Can you work these out from the model? Positions are in its coordinate system, mm. A direction names the side the tool comes from. Round coordinates to 2 decimals unless told otherwise and drop trailing zeros. Loops run counter-clockwise (first coordinate to the right, second up) from the corner with the lowest first, then second, coordinate; pieces in that order, holes last. Notation, with made-up numbers: M -25,80.25 L -17,80.25 A14 cw -17,89.25 Z; hole C 74,-2.5 d2. An arc over 180 degrees is marked long. Return JSON: item names as keys, results as strings.
```python
from build123d import *

# Parameters (mm, degrees)
SKETCH_1_R          = 1.55
EXTRUDE_1_DEPTH     = 3
CUT_EXTRUDE_1_DEPTH = 1
CHAMFER_1_SIZE      = 0.3


with BuildPart() as part:
    # 草图1 → 凸台-拉伸1 (new body)
    with BuildSketch(Plane(origin=(0, 0, 0), x_dir=(-1, 0, 0), z_dir=(0, 0, -1))):
        with BuildLine():
            Line((-47.519320255, 26.959319012), (-50.6992, 14.4996))
            Line((-50.6992, 14.4996), (-50.6992, 10.0003))
            Line((-50.6992, 10.0003), (-53.6992, 10.0003))
            Line((-53.6992, 10.0003), (-53.6992, 0))
            Line((-53.6992, 0), (-50.6992, 0))
            Line((-50.6992, 0), (-50.6992, -1.5007))
            Line((-50.6992, -1.5007), (-49.2382, -1.5007))
            Line((-49.2382, -1.5007), (-49.2382, -4.5007))
            Line((-49.2382, -4.5007), (-40.2392, -4.5007))
            Line((-40.2392, -4.5007), (-40.2392, -1.4993))
            Line((-40.2392, -1.4993), (-34.2002, -1.4993))
            Line((-34.2002, -1.4993), (-34.2002, 1.0005))
            Line((-34.2002, 1.0005), (-19.2003, 1.0005))
            Line((-19.2003, 1.0005), (-19.2003, -1.4993))
            Line((-19.2003, -1.4993), (-11.7217, -1.4993))
            Line((-11.7217, -1.4993), (-11.7217, -4.5007))
            Line((-11.7217, -4.5007), (-4.3215, -4.5007))
            Line((-4.3215, -4.5007), (-4.3215, -1.5007))
            Line((-4.3215, -1.5007), (-3, -1.5007))
            Line((-3, -1.5007), (-3, 0))
            Line((-3, 0), (0, 0))
            Line((0, 0), (0, 10.0003))
            Line((0, 10.0003), (-3, 10.0003))
            Line((-3, 10.0003), (-3, 14.4996))
            Line((-3, 14.4996), (-26.543543046, 20.807804388))
            ThreePointArc((-26.543543046, 20.807804388), (-32.65852857, 22.990550509), (-36.548909006, 28.188854909))
            ThreePointArc((-36.548909006, 28.188854909), (-38.379715818, 30.572322748), (-41.246222879, 31.4756))
            Line((-41.246222879, 31.4756), (-41.70566582, 31.4756))
            ThreePointArc((-41.70566582, 31.4756), (-45.386541118, 30.213865193), (-47.519320255, 26.959319012))
        make_face()
        with Locations(Location((-41.6992, 25.49975, 0), (0, 0, 180))):
            Circle(SKETCH_1_R, mode=Mode.SUBTRACT)
    extrude(amount=-EXTRUDE_1_DEPTH)

    # 草图2 → 切除-拉伸1 (cut)
    with BuildSketch(Plane.XY.offset(3)):
        Polygon((43.327916651, 19.948770062), (43.975052068, 19.948770062), (43.975052068, 16.448770062), (43.660949504, 16.448770062), (43.660949504, 19.589795703), (43.122487965, 19.589795703), align=None)
        Polygon((46.020224344, 19.948770062), (46.66735976, 19.948770062), (46.66735976, 16.448770062), (46.353257196, 16.448770062), (46.353257196, 19.589795703), (45.814795658, 19.589795703), align=None)
    extrude(amount=-CUT_EXTRUDE_1_DEPTH, mode=Mode.SUBTRACT)

    # 倒角1
    chamfer_1_edges = [part.edges().sort_by_distance(p)[0] for p in [
        (40.1492, 25.49975, 3),
        (40.1492, 25.49975, 0),
    ]]
    chamfer(chamfer_1_edges, length=CHAMFER_1_SIZE)


solid = part.part
```
Q1. On a 3-axis mill with a long thin cutter (end or side, diameter ignored), from which of +Z, -Z, +X, -X, +Y, -Y can I reach the whole of each face in a straight line? I mean faces 1 (the flat face through (50, -1.501, 1)), 2 (the flat face through (53.699, 5, 1)), 3 (the flat face through (40.239, -3, 1)), 4 (the flat face through (4.322, -3, 1)). Say none if no direction works.
Results:
{"face 1": "+Z, -Z, +X, -Y", "face 2": "+Z, -Z, +X, +Y, -Y", "face 3": "+Z, -Z, -Y", "face 4": "+Z, -Z, -X, -Y"}
Q2. If I drill on line 1 along X through (y, z) = (-3, 0.9); line 2 along X through (y, z) = (12, 1.3); line 3 along Y through (x, z) = (51.5, 0.8), over which ranges is the centre line in solid material (lowest first)?
Results:
{"line 1": "x = 4.32 to 11.72, 40.24 to 49.24", "line 2": "x = 3 to 50.7", "line 3": "y = 0 to 10"}
Q3. Suppose I cut it at C-C, the plane x = 13.5. Please give me the cut outline in (y, z), plus the area to 3 significant figures.
Results:
{"outline": "M -1.5,0 L 17.31,0 L 17.31,3 L -1.5,3 Z", "area": "56.4 mm2"}
Q4. Thinking about a two-plate mould opening in Y: for faces 5 (the flat face through (19.2, 0, 1)), 6 (the flat face through (43.975, 18.2, 2.5)), 7 (the cylindrical face through (43.131, 26.093, 1.483)), 8 (the flat face through (16, -1.499, 1)), which applies, pulls with the +Y half, pulls with the -Y half, needs draft (parallel to the pull), parting line crosses it, or undercut?
Results:
{"face 5": "needs draft", "face 6": "undercut", "face 7": "undercut", "face 8": "pulls with the -Y half"}
Q5. Suppose I cut it at B-B, the plane x = 6.5. Please give me the cut outline in (y, z).
Results:
{"outline": "M -4.5,0 L 15.44,0 L 15.44,3 L -4.5,3 Z"}
Q6. I'm going to push flat-ended pins straight in: pin 1 Ø1.5 at (x, z) = (52.5, 2) entering from -Y; pin 2 Ø1.5 at (y, z) = (-3, 1) entering from +X; pin 3 Ø1.5 at (x, z) = (52, 2) entering from +Y. Where does each tip first touch, or does it pass through?
Results:
{"pin 1": "stops at y = 0", "pin 2": "stops at x = 49.24", "pin 3": "stops at y = 10"}
